Job drawing, mm, ordinate dimensions from the low corner. One solid piece. A direction names the side the tool comes from. Round coordinates to 2 decimals unless told otherwise and drop trailing zeros. Write each loop counter-clockwise with the first axis right and the second up, starting at its lowest first coordinate (ties: lowest second). Pieces come first, ordered by that corner, then holes.
1) Saw through at B-B (y = 3.25). Write the cut outline in (x, z), plus the area to 3 significant figures.
2) Saw through at D-D (z = 16.5). Write the cut outline in (x, y).
3) Which spindle directions (+Z, -Z, +X, -X, +Y, -Y) get a long thin tool onto all of the face, cutting with end or side? Do the marked faces 1 and 2. Say none if no direction does.
4) Saw through at A-A (y = 8.5). Write the cut outline in (x, z), plus the area to 3 significant figures.
5) Wall check: probe 1 along Z at (x, y) = (51, 5.5); probe 2 along Z at (x, y) = (14, 8.25); probe 3 along Z at (x, y) = (6, 6.25). Give the ranges that are in metal, low to high.
6) Saw through at C-C (x = 51). Write the cut outline in (y, z).
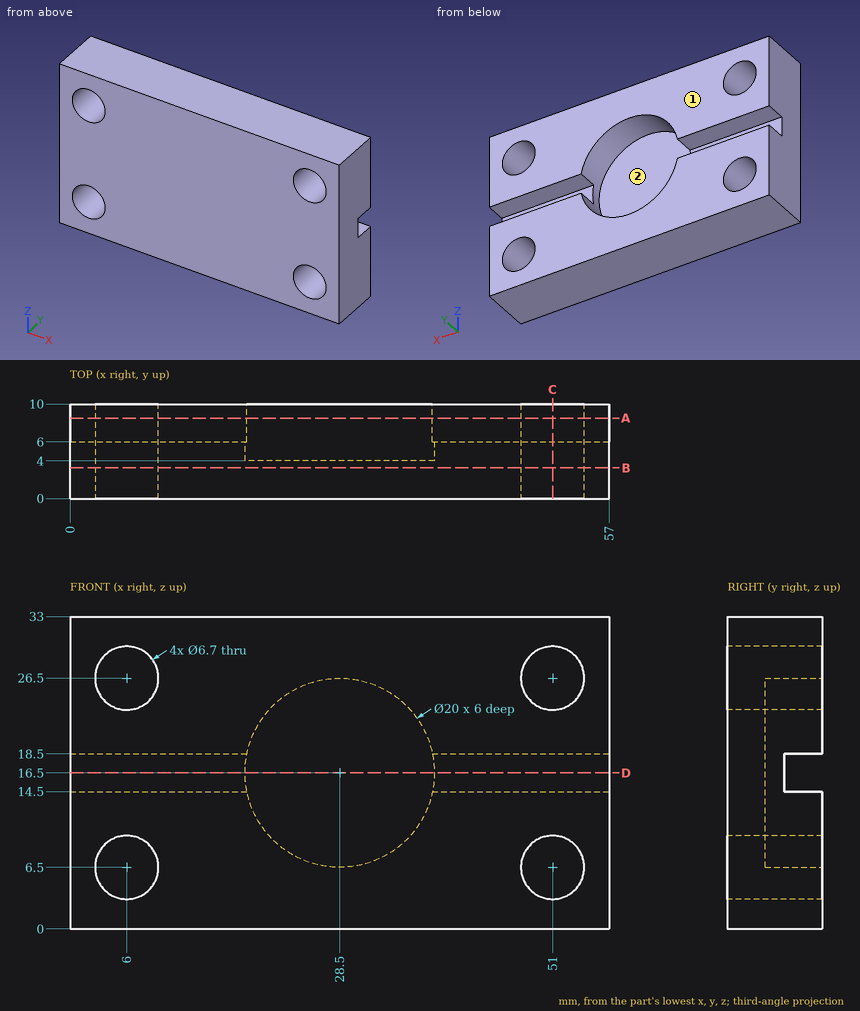
Evaluation:
1. outline: (0, 0) - (57, 0) - (57, 33) - (0, 33) - close; hole circle Ø6.7 at (6, 6.5); hole circle Ø6.7 at (6, 26.5); hole circle Ø6.7 at (51, 6.5); hole circle Ø6.7 at (51, 26.5)
1. area: 1,740 mm2
2. outline: (0, 0) - (57, 0) - (57, 6) - (38.5, 6) - (38.5, 4) - (18.5, 4) - (18.5, 6) - (0, 6) - close
3. face 1: +Z, -Z, +X, -X, +Y
3. face 2: +Y
4. outline: (0, 0) - (57, 0) - (57, 14.5) - (38.3, 14.5) arc R10 cw to (18.7, 14.5) - (0, 14.5) - close; (0, 18.5) - (18.7, 18.5) arc R10 cw to (38.3, 18.5) - (57, 18.5) - (57, 33) - (0, 33) - close; hole circle Ø6.7 at (6, 6.5); hole circle Ø6.7 at (6, 26.5); hole circle Ø6.7 at (51, 6.5); hole circle Ø6.7 at (51, 26.5)
4. area: 1,280 mm2
5. probe 1: z = 0 to 3.15, 9.85 to 23.15, 29.85 to 33
5. probe 2: z = 0 to 14.5, 18.5 to 33
5. probe 3: z = 0 to 3.15, 9.85 to 14.5, 18.5 to 23.15, 29.85 to 33
6. outline: (0, 0) - (10, 0) - (10, 3.15) - (0, 3.15) - close; (0, 9.85) - (10, 9.85) - (10, 14.5) - (6, 14.5) - (6, 18.5) - (10, 18.5) - (10, 23.15) - (0, 23.15) - close; (0, 29.85) - (10, 29.85) - (10, 33) - (0, 33) - close
